Can you work these out from the model? Positions are in its coordinate system, mm. Face numbers are marked on the shaded views. A direction names the side the tool comes from. Coordinates: 2 decimals unless noted, no trailing zeros. Order: outer loops, then holes, each group sorted by start corner. A loop starts at its lowest first (then second) coordinate and runs counter-clockwise, first axis right, second up. Notation, with made-up numbers: M 48,-22.5 L 79,-22.5 A23 ccw 79,-10.5 Z; hole C -17.5,10 d8. An arc over 180 degrees is marked long. Answer as CSV lines item,"result". Start each with the question number.
1. If we section it at A-A (x = 9.5): List the corners of the cut face in (y, z) for me, plus the area to 4 significant figures.
2. Will these pins go through, and if not, where does the flat tip stop? pin 1 (3 mm diameter, centred on x = 1, z = 5, fed in from -Y); pin 2 (6 mm diameter, centred on y = -15, z = 3, fed in from -X); pin 3 (1.5 mm diameter, centred on x = 0.5, y = 10.5, fed in from -Z).
3. If we section it at C-C (z = 1): List the corners of the cut face in (x, y) for me.
4. If we mould it in two halves opening along X, with no side actions, what happens to the marked faces 4, 5 and 6? For each: released by +X, released by -X, zero draft, split by the parting line, or undercut.
5. On a 3-axis mill with a long thin cutter (end or side, diameter ignored), from which of +Z, -Z, +X, -X, +Y, -Y can I reach the whole of each face in a straight line? I mean the marked faces 1, 2 and 3. Say none if no direction works.
6. If we section it at B-B (y = 1): List the corners of the cut face in (x, z) for me, plus the area to 3 significant figures.
7. I need wall thicknesses on line 1 along Y through (x, z) = (-13, 7); line 2 along X through (y, z) = (4, 3.75); line 3 along X through (y, z) = (-15, 2.75). Which ranges of each line are inside material? Lowest first, please. Write a range as from..to.
8. If we section it at D-D (z = 9.25): List the corners of the cut face in (x, y) for me.
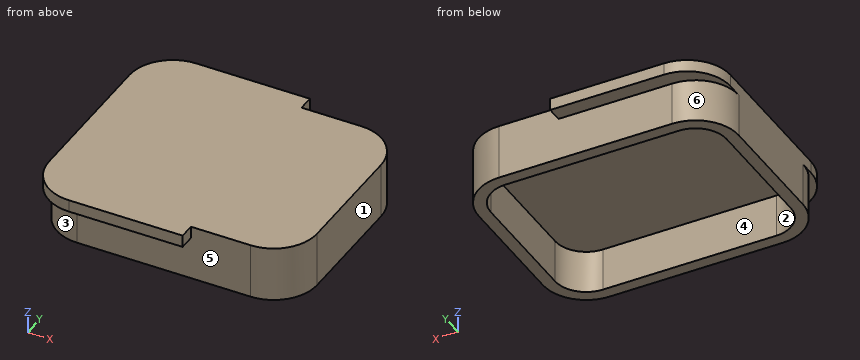
```python
from build123d import *

# Parameters (mm, degrees)
F1_DEPTH     = 10.25
F3_DEPTH     = 2.25
F4_T         = 2.25
F4_T3_DEPTH  = 25.5
F4_T5_DEPTH  = 6.75
F4_T8_ANGLE  = 90.000000001
F4_T10_ANGLE = 90.000000001


# Not quite as in the source:
# - a shell that OpenCascade refuses in one call is made with other operations: the cavity is built on its own and cut out


with BuildPart() as f1:
    # F0 (on Top) → F1 (new body)
    with BuildSketch(Plane.XY):
        with BuildLine():
            Line((16, 19), (-16, 19))
            ThreePointArc((-16, 19), (-21.6568542495, 16.6568542495), (-24, 11))
            Line((-24, 11), (-24, -11))
            ThreePointArc((-24, -11), (-21.6568542495, -16.6568542495), (-16, -19))
            Line((-16, -19), (16, -19))
            ThreePointArc((16, -19), (21.6568542495, -16.6568542495), (24, -11))
            Line((24, -11), (24, 11))
            ThreePointArc((24, 11), (21.6568542495, 16.6568542495), (16, 19))
        make_face()
    extrude(amount=F1_DEPTH)

    # F2 (on face) → F3 (join)
    with BuildSketch(Plane.XY.offset(10.25)):
        with BuildLine():
            Line((5, 21.85), (-16, 21.85))
            ThreePointArc((-16, 21.85), (-21.6568542495, 19.5068542495), (-24, 13.85))
            Line((-24, 13.85), (-24, -13.85))
            ThreePointArc((-24, -13.85), (-21.6568542495, -19.5068542495), (-16, -21.85))
            Line((-16, -21.85), (5, -21.85))
            Line((5, -21.85), (5, 21.85))
        make_face()
    extrude(amount=-F3_DEPTH)

    # F4: shell of thickness 2.25, made by hand


with BuildPart() as f4_core1:
    # F4_t2: copy of F1
    add(f1.part)

    # the walls: a layer under each face that stays
    f4_faces = [f4_core1.faces().sort_by_distance(p)[0] for p in [
        (0, 19, 5.125),
        (21.6568542495, 16.6568542495, 5.125),
        (24, 0, 5.125),
        (21.6568542495, -16.6568542495, 5.125),
        (0, -19, 5.125),
        (-21.6568542495, -16.6568542495, 4),
        (-24, 0, 5.125),
        (-21.6568542495, -19.5068542495, 9.125),
        (-5.5, -21.85, 9.125),
        (-21.6568542495, 19.5068542495, 9.125),
        (-5.5, 21.85, 9.125),
        (-19.1666666667, -20.0416666667, 8),
        (5, -20.425, 9.125),
        (0, 0, 10.25),
        (5, 20.425, 9.125),
        (-19.1666666667, 20.0416666667, 8),
        (-21.6568542495, 16.6568542495, 4),
    ]]
    thicken(f4_faces, amount=-F4_T, mode=Mode.SUBTRACT)

    # F4_s4 → F4_t3 (cut)
    with BuildSketch(Plane.YZ.offset(-18.25)):
        Polygon((19.0225, 7.9775), (16.75, 8), (16.75, 10.25), (19, 10.25), align=None)
        Polygon((-19.0225, 7.9775), (-16.75, 8), (-16.75, 10.25), (-19, 10.25), align=None)
    extrude(amount=F4_T3_DEPTH, mode=Mode.SUBTRACT)

    # F4_s6 → F4_t5 (cut)
    with BuildSketch(Plane.XY.offset(5.75)):
        Polygon((5.0225, 19.0225), (5, 16.75), (2.75, 16.75), (2.75, 19), align=None)
        Polygon((5.0225, -19.0225), (5, -16.75), (2.75, -16.75), (2.75, -19), align=None)
    extrude(amount=F4_T5_DEPTH, mode=Mode.SUBTRACT)

    # F4_s7 → F4_t8 (revolve, cut)
    with BuildSketch(Plane.YZ.offset(-16)):
        Polygon((-19.0225, 7.9775), (-16.75, 8), (-16.75, 10.25), (-19, 10.25), align=None)
    revolve(axis=Axis((-16, -11, 8), (0, 0, -1)), revolution_arc=F4_T8_ANGLE, mode=Mode.SUBTRACT)

    # F4_s9 → F4_t10 (revolve, cut)
    with BuildSketch(Plane.XZ.offset(-11)):
        Polygon((-24.0225, 7.9775), (-24, 10.25), (-21.75, 10.25), (-21.75, 8), align=None)
    revolve(axis=Axis((-16, 11, 8), (0, 0, -1)), revolution_arc=F4_T10_ANGLE, mode=Mode.SUBTRACT)


with BuildPart() as f1_1:
    add(f1.part)

    # what is left inside the walls is the cavity
    f4_cavity = [f4_core1.part.solids().sort_by_distance(p)[0] for p in [
        (0, -5.583333, 7.9775),
    ]]
    add(f4_cavity, mode=Mode.SUBTRACT)


solid = f1_1.part
```
Solved:
1,outline,"M -19,0 L -16.75,0 L -16.75,8 L 16.75,8 L 16.75,0 L 19,0 L 19,10.25 L -19,10.25 Z"
1,area,"121.5 mm²"
2,pin 1,"y = -19"
2,pin 2,"x = -23.94"
2,pin 3,"z = 8"
3,outline,"M -24,-11 A8 ccw -16,-19 L 16,-19 A8 ccw 24,-11 L 24,11 A8 ccw 16,19 L -16,19 A8 ccw -24,11 Z; hole M -21.75,-11 A5.75 ccw -16,-16.75 L 16,-16.75 A5.75 ccw 21.75,-11 L 21.75,11 A5.75 ccw 16,16.75 L -16,16.75 A5.75 ccw -21.75,11 Z"
4,face 4,"undercut"
4,face 5,"zero draft"
4,face 6,"released by -X"
5,face 1,"+Z, -Z, +X, +Y, -Y"
5,face 2,"-Z"
5,face 3,"-Z, -X, -Y"
6,outline,"M -24,0 L -21.75,0 L -21.75,8 L 21.75,8 L 21.75,0 L 24,0 L 24,10.25 L -24,10.25 Z"
6,area,"144 mm²"
7,line 1,"-19..-16.75, 16.75..19"
7,line 2,"-24..-21.75, 21.75..24"
7,line 3,"-22.93..-20.13, 20.13..22.93"
8,outline,"M -24,-13.85 A8 ccw -16,-21.85 L 5,-21.85 L 5,-19 L 16,-19 A8 ccw 24,-11 L 24,11 A8 ccw 16,19 L 5,19 L 5,21.85 L -16,21.85 A8 ccw -24,13.85 Z"
